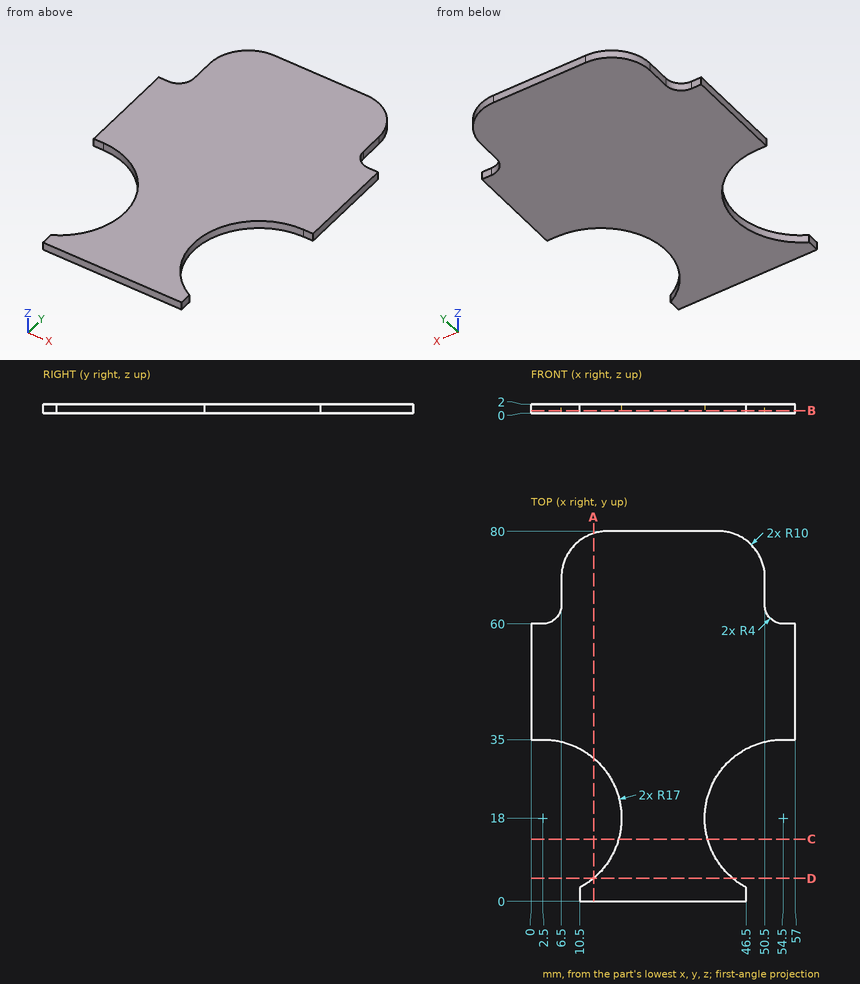
Job drawing, mm, ordinate dimensions from the low corner. One solid piece. Give positions to 0.01 mm unless a question says otherwise; leave off trailing zeros. Order: outer loops, then holes, each group sorted by start corner. A loop starts at its lowest first (then second) coordinate and runs counter-clockwise, first axis right, second up. Notation, with made-up numbers: M 9.25,5.5 L 27.25,5.5 A19 ccw 27.25,39.5 Z; hole C 88,-27 d5. An arc over 180 degrees is marked long. Put each result on its own line as item: value. Start each with the question number.
(1) Pin check, flat tips, straight feed: pin 1 Ø0.6 at (y, z) = (68.5, 1.5) entering from +X; pin 2 Ø0.6 at (y, z) = (2, 1) entering from -X. Stop position of each tip, or through.
(2) Band-saw the part on A-A on x = 13.5. Give the cut face in (y, z).
(3) Drill centre lines: L1, parallel to Y at x = 45.5, z = 0.6; L2, parallel to X at y = 15, z = 1.75; L3, parallel to Y at x = 11, z = 0.9. Where is each one in solid material? Low to high. Write a range as [from, to].
(4) Band-saw the part on C-C on y = 13.5. Give the cut face in (x, z).
(5) Band-saw the part on B-B on z = 0.55. Give the cut face in (x, y), then the cut area to 3 significant figures.
(6) Band-saw the part on D-D on y = 5. Give the cut face in (x, z) (1 decimal).
Results below:
1. pin 1: stops at x = 50.5
1. pin 2: stops at x = 10.5
2. outline: M 0,0 L 5.04,0 L 5.04,2 L 0,2 Z; M 30.96,0 L 79.54,0 L 79.54,2 L 30.96,2 Z
3. L1: y = [0, 3.58], [32.42, 78.66]
3. L2: x = [19.23, 37.77]
3. L3: y = [0, 3.28], [32.72, 78.35]
4. outline: M 18.89,0 L 38.11,0 L 38.11,2 L 18.89,2 Z
5. outline: M 0,35 L 2.5,35 A17 cw 10.5,3 L 10.5,0 L 46.5,0 L 46.5,3 A17 cw 54.5,35 L 57,35 L 57,60 L 54.5,60 A4 cw 50.5,64 L 50.5,70 A10 ccw 40.5,80 L 16.5,80 A10 ccw 6.5,70 L 6.5,64 A4 cw 2.5,60 L 0,60 Z
5. area: 3,150 mm2
6. outline: M 13.5,0 L 43.5,0 L 43.5,2 L 13.5,2 Z
